```python
from build123d import *

# Parameters (mm, degrees)
BOSS_EXTRUDE1_DEPTH     = 9.525
F_1_4_20_TAPPED_HOLE1_D = 5.1054


with BuildPart() as part:
    # Sketch2 → Boss-Extrude1 (new body)
    with BuildSketch(Plane.XY):
        with BuildLine():
            Line((0, -63.5), (63.5, -63.5))
            Line((63.5, -63.5), (63.5, -48.26))
            Line((63.5, -48.26), (0, -48.26))
            ThreePointArc((0, -48.26), (-44.110630078, -19.577535956), (-35.788539013, 32.376041687))
            ThreePointArc((-35.788539013, 32.376041687), (-35.1329407, 34.143563747), (-35.876095105, 35.876095105))
            Line((-35.876095105, 35.876095105), (-43.067795393, 43.067795393))
            ThreePointArc((-43.067795393, 43.067795393), (-44.916774776, 43.811192654), (-46.733173559, 42.991400176))
            ThreePointArc((-46.733173559, 42.991400176), (-58.147243749, -25.517602639), (0, -63.5))
        make_face()
    extrude(amount=BOSS_EXTRUDE1_DEPTH)

    # 1/4-20 Tapped Hole1 (through all)
    with Locations(Plane.XY.offset(9.525)):
        with Locations((8.89, -55.88), (41.91, -55.88)):
            Hole(F_1_4_20_TAPPED_HOLE1_D / 2)


solid = part.part
```
Check sheet for the modelled part. Datum: model origin and axes. Units: mm. A direction names the side the tool comes from. Round coordinates to 2 decimals unless told otherwise and drop trailing zeros. Loops run counter-clockwise (first coordinate to the right, second up) from the corner with the lowest first, then second, coordinate; pieces in that order, holes last. Notation, with made-up numbers: (26.5, 13.25) - (74.5, 13.25) arc R4 ccw to (74.5, 17.25) - close; hole circle Ø6 at (88.25, 68.25). An arc over 180 degrees is marked (long way). Write item = value, one per line. Start each with the question number.
Q1. Section check D-D (x = 28.5). Record the boundary of the cut face in (y, z) (3 decimals).
Q2. Depth check by flat-ended pin: P1, Ø2, axis at x = 25.5, z = 6.5, coming from the +Y side; P2, Ø3, axis at x = 8.89, y = -55.88, coming from the -Z side; P3, Ø1.5, axis at y = -9, z = 3.5, coming from the +X side; P4, Ø6.5, axis at x = 41.91, y = -55.88, coming from the +Z side (3 decimals). Enter the tip coordinate at first touch or a pass-through.
Q3. Section check C-C (z = 4). Record the boundary of the cut face in (x, y), plus the area to 3 significant figures.
Q4. Section check B-B (y = -55.88). Record the boundary of the cut face in (x, z) (3 decimals), plus the area to 3 significant figures.
Q5. Thickness scan on L1, parallel to Y at x = 8.89, z = 7.75; L2, parallel to Y at x = 3, z = 7.5; L3, parallel to Y at x = 41, z = 2.75. Record the ranges inside material, lowest first.
Q6. Section check A-A (x = 8.89). Record the boundary of the cut face in (y, z) (3 decimals), plus the area to 3 significant figures.
Q7. Release check for a two-part mould opening along Y. For faces 1 (the face through (42.463, -58.372, 4.696)), 2 (the face through (-19, -45, 0)), 3 (the face through (-39, 39, 5)), 4 (the face through (-58.553, -24.572, 4.696)) record: pulls with the +Y half, pulls with the -Y half, needs draft (parallel to the pull), parting line crosses it, or undercut.
Q8. Access from +Z, -Z, +X, -X, +Y, -Y to the whole of each face (thin tool, end or side, straight path). Record for faces 5 (the face through (32, -48.26, 5)), 6 (the face through (9.443, -58.372, 4.696)).
Derived:
q1.outline = (-63.5, 0) - (-48.26, 0) - (-48.26, 9.525) - (-63.5, 9.525) - close
q2.P1 = -48.26
q2.P2 = through
q2.P3 = -47.26
q2.P4 = 9.525
q3.outline = (-46.73, 42.99) arc R63.5 ccw to (0, -63.5) - (63.5, -63.5) - (63.5, -48.26) - (0, -48.26) arc R48.26 cw to (-35.79, 32.38) arc R2.54 ccw to (-35.88, 35.88) - (-43.07, 43.07) arc R2.54 ccw to start; hole circle Ø5.11 at (8.89, -55.88); hole circle Ø5.11 at (41.91, -55.88)
q3.area = 2,930 mm^2
q4.outline = (-30.161, 0) - (6.337, 0) - (6.337, 9.525) - (-30.161, 9.525) - close; (11.443, 0) - (39.357, 0) - (39.357, 9.525) - (11.443, 9.525) - close; (44.463, 0) - (63.5, 0) - (63.5, 9.525) - (44.463, 9.525) - close
q4.area = 795 mm^2
q5.L1 = -63.5 to -58.43, -53.33 to -48.26
q5.L2 = -63.5 to -48.26
q5.L3 = -63.5 to -58.26, -53.5 to -48.26
q6.outline = (-63.5, 0) - (-58.433, 0) - (-58.433, 9.525) - (-63.5, 9.525) - close; (-53.327, 0) - (-48.26, 0) - (-48.26, 9.525) - (-53.327, 9.525) - close
q6.area = 96.5 mm^2
q7.face_1 = undercut
q7.face_2 = needs draft
q7.face_3 = pulls with the +Y half
q7.face_4 = parting line crosses it
q8.face_5 = +Z, -Z, +X, +Y
q8.face_6 = +Z, -Z
